from build123d import *

# Parameters (mm, degrees)
SKETCH3_W           = 140
SKETCH3_H           = 85
BOSS_EXTRUDE1_DEPTH = 3
SKETCH4_R           = 1.6
CUT_EXTRUDE1_DEPTH  = 3
FILLET1_R           = 10
FILLET2_R           = 10
FILLET3_R           = 10
FILLET4_R           = 10
SKETCH7_R           = 1
SKETCH7_W           = 11.6
SKETCH7_H           = 22.5
CUT_EXTRUDE4_DEPTH  = 3


with BuildPart() as part:
    # Sketch3 → Boss-Extrude1 (new body)
    with BuildSketch(Plane(origin=(0, 0, 0), x_dir=(1, 0, 0), z_dir=(0, 1, 0))):
        Rectangle(SKETCH3_W, SKETCH3_H)
    extrude(amount=BOSS_EXTRUDE1_DEPTH)

    # Sketch4 → Cut-Extrude1 (cut)
    with BuildSketch(Plane(origin=(0, 3, 0), x_dir=(1, 0, 0), z_dir=(0, 1, 0))):
        with Locations((-43.4, 15.8)):
            Circle(SKETCH4_R)
        with Locations((7.4, 0.5)):
            Circle(SKETCH4_R)
        with Locations((-45, -32.5)):
            Circle(SKETCH4_R)
        with Locations((7.4, -27.4)):
            Circle(SKETCH4_R)
    extrude(amount=-CUT_EXTRUDE1_DEPTH, mode=Mode.SUBTRACT)

    # Fillet1
    fillet1_edges = [part.edges().sort_by_distance(p)[0] for p in [
        (-70, 1.5, 42.5),
    ]]
    fillet(fillet1_edges, radius=FILLET1_R)

    # Fillet2
    fillet2_edges = [part.edges().sort_by_distance(p)[0] for p in [
        (-70, 1.5, -42.5),
    ]]
    fillet(fillet2_edges, radius=FILLET2_R)

    # Fillet3
    fillet3_edges = [part.edges().sort_by_distance(p)[0] for p in [
        (70, 1.5, -42.5),
    ]]
    fillet(fillet3_edges, radius=FILLET3_R)

    # Fillet4
    fillet4_edges = [part.edges().sort_by_distance(p)[0] for p in [
        (70, 1.5, 42.5),
    ]]
    fillet(fillet4_edges, radius=FILLET4_R)

    # Sketch7 → Cut-Extrude4 (cut)
    with BuildSketch(Plane(origin=(0, 3, 0), x_dir=(1, 0, 0), z_dir=(0, 1, 0))):
        with Locations((54.2, -31.25)):
            Circle(SKETCH7_R)
        with Locations((54.2, -3.75)):
            Circle(SKETCH7_R)
        with Locations((54.2, -17.5)):
            Rectangle(SKETCH7_W, SKETCH7_H)
    extrude(amount=-CUT_EXTRUDE4_DEPTH, mode=Mode.SUBTRACT)


solid = part.part
CAD build for the part. Positions are in the model's coordinates, mm. A direction names the side the tool comes from. Coordinates: 2 decimals unless noted, no trailing zeros. Loops run counter-clockwise (first coordinate to the right, second up) from the corner with the lowest first, then second, coordinate; pieces in that order, holes last. Notation, with made-up numbers: (15.25, -40) - (43.25, -40) arc R29 cw to (43.25, -11) - close; hole circle Ø8 at (-34, 7). An arc over 180 degrees is marked (long way). Use one line per item in the form item = value. Start each with the question number.
1) Drill centre lines: L1, parallel to Z at x = 54.2, y = 2.25; L2, parallel to Z at x = 7.4, y = 2.15; L3, parallel to X at y = 1.75, z = 8. Where is each one in solid material? Low to high. Write a range as from..to.
2) Tool access for faces 4 (the face through (54, 2, 6.25)), 5 (the face through (-1, 1, 42.5)): list every direction of +Z, -Z, +X, -X, +Y, -Y with a clear straight run to the whole face (end or side of a thin tool).
3) Band-saw the part on B-B (x = 7.4). Give the cut face in (y, z), and give its area (3 significant figures).
4) Flat gauge pin, fed straight in: pin 1 (2.5 mm diameter, centred on x = 7.4, z = 27.4, fed in from -Y). Where does the tip first touch, or does it go through?
5) Two-plate mould, pull along Z, no slides. Class faces 1 (the face through (-1, 3, -1)), 2 (the face through (-43.75, 1.52, -14.24)), 3 (the face through (-67.15, 1.52, -39.49)): +Z half, -Z half, draft (parallel to the pull), parting line (faces both ways), or undercut.
6) Band-saw the part on A-A (z = 27.4). Give the cut face in (x, y), and give its area (3 significant figures).
7) Band-saw the part on C-C (y = 1.75). Give the cut face in (x, z), and give its area (3 significant figures).
Check values:
q1.L1 = -42.5..2.75, 4.75..6.25, 28.75..30.25, 32.25..42.5
q1.L2 = -42.5..-2.1, 1.1..25.8, 29..42.5
q1.L3 = -70..48.4, 60..70
q2.face_4 = +Y, -Y
q2.face_5 = +Z, +X, -X, +Y, -Y
q3.outline = (0, -42.5) - (3, -42.5) - (3, -2.1) - (0, -2.1) - close; (0, 1.1) - (3, 1.1) - (3, 25.8) - (0, 25.8) - close; (0, 29) - (3, 29) - (3, 42.5) - (0, 42.5) - close
q3.area = 236 mm2
q4.pin_1 = through
q5.face_1 = draft
q5.face_2 = undercut
q5.face_3 = -Z half
q6.outline = (-70, 0) - (5.8, 0) - (5.8, 3) - (-70, 3) - close; (9, 0) - (48.4, 0) - (48.4, 3) - (9, 3) - close; (60, 0) - (70, 0) - (70, 3) - (60, 3) - close
q6.area = 376 mm2
q7.outline = (-70, -32.5) arc R10 ccw to (-60, -42.5) - (60, -42.5) arc R10 ccw to (70, -32.5) - (70, 32.5) arc R10 ccw to (60, 42.5) - (-60, 42.5) arc R10 ccw to (-70, 32.5) - close; hole circle Ø3.2 at (-45, 32.5); hole circle Ø3.2 at (-43.4, -15.8); hole circle Ø3.2 at (7.4, -0.5); hole circle Ø3.2 at (7.4, 27.4); hole (48.4, 6.25) - (60, 6.25) - (60, 28.75) - (48.4, 28.75) - close; hole circle Ø2 at (54.2, 3.75); hole circle Ø2 at (54.2, 31.25)
q7.area = 11,500 mm2
